Geometry: final body of the model. Coordinates: model frame, mm. A direction names the side the tool comes from. Coordinates: 2 decimals unless noted, no trailing zeros. Loops run counter-clockwise (first coordinate to the right, second up) from the corner with the lowest first, then second, coordinate; pieces in that order, holes last. Notation, with made-up numbers: M 23,42 L 34,42 A8 ccw 34,52 Z; hole C 64.25,-30 d3. An arc over 180 degrees is marked long. Write each question's results on one line, items separated by ' | '. Start each with the question number.
from build123d import *

# Parameters (mm, degrees)
F1_DEPTH  = 29
F0_W      = 28.9777747887
F0_H      = 95.25
F2_DEPTH  = 29
F5_DEPTH  = 3
F6_R      = 2.5
F7_D      = 3.2639
F10_R     = 2.5
F9_W      = 60
F9_H      = 26
F11_DEPTH = 97.505434954
F16_DEPTH = 0.5
F19_DEPTH = 0.5
F22_DEPTH = 0.5
F23_D     = 6.7564


# Not quite as in the source:
# - a feature names something its author has since deleted; it is built from what else it names


with BuildPart() as f1:
    # F0 (on Front) → F1 (new body)
    with BuildSketch(Plane.XZ):
        Polygon((28.9777747887, 7.7645713531), (0, 0), (28.9777747887, 0), align=None)
    extrude(amount=F1_DEPTH)

    # F0 (on Front) → F2 (join)
    with BuildSketch(Plane.XZ):
        Polygon((28.9777747887, 7.7645713531), (0, 0), (28.9777747887, 0), align=None)
        with Locations((14.4888873943, -47.625)):
            Rectangle(F0_W, F0_H)
    extrude(amount=F2_DEPTH)

    # F4 (on face) → F5 (join)
    with BuildSketch(Plane(origin=(0, 0, -95.25), x_dir=(1, 0, 0), z_dir=(0, 0, -1))):
        Polygon((0, 29), (14.4888873943, 29), (28.9777747887, 29), (28.9777747887, 34), (0, 34), align=None)
        Polygon((28.9777747887, 0), (14.4888873943, 0), (0, 0), (0, -5), (28.9777747887, -5), align=None)
    extrude(amount=-F5_DEPTH)

    # F6
    f6_edges = [f1.edges().sort_by_distance(p)[0] for p in [
        (28.977775, -34, -93.75),
        (0, -34, -93.75),
    ]]
    fillet(f6_edges, radius=F6_R)

    # F7 (through all)
    with Locations(Plane(origin=(0, 0, -95.25), x_dir=(1, 0, 0), z_dir=(0, 0, -1))):
        with Locations((2.5, 31.5), (14.4888873943, 31.5), (26.4777747887, 31.5), (2.5, -2.5), (14.4888873943, -2.5), (26.4777747887, -2.5)):
            Hole(F7_D / 2)

    # F10
    f10_edges = [f1.edges().sort_by_distance(p)[0] for p in [
        (28.977775, 5, -93.75),
        (0, 5, -93.75),
    ]]
    fillet(f10_edges, radius=F10_R)

    # F9 (on offset) → F11 (cut, through all)
    with BuildSketch(Plane(origin=(0.5176380902, 0, -1.9318516526), x_dir=(0.9659258263, 0, 0.2588190451), z_dir=(-0.2588190451, 0, 0.9659258263))):
        with Locations((-0.5358983849, -14.5)):
            Rectangle(F9_W, F9_H)
    extrude(amount=-F11_DEPTH, mode=Mode.SUBTRACT)

    # F15 (on plane+point) → F16 (join, symmetric)
    with BuildSketch(Plane.YZ.offset(20.4833310915)):
        Polygon((-29, -92.25), (-29, 5.4884920243), (-34, -92.25), align=None)
        Polygon((5, -92.25), (0, 5.4884920243), (0, -92.25), align=None)
    extrude(amount=F16_DEPTH, both=True)

    # F18 (on plane+point) → F19 (join, symmetric)
    with BuildSketch(Plane.YZ.offset(8.4944436972)):
        Polygon((5, -92.25), (0, 2.2760793288), (0, -92.25), align=None)
        Polygon((-34, -92.25), (-29, -92.25), (-29, 2.2760793288), align=None)
    extrude(amount=F19_DEPTH, both=True)

    # F21 (on plane+point) → F22 (join, symmetric)
    with BuildSketch(Plane.YZ.offset(14.4888873943)):
        Polygon((-27.5, 1.8117333157), (-27.5, -95.25), (-19.5, 1.8117333157), align=None)
        Polygon((-1.5, 1.8117333157), (-9.5, 1.8117333157), (-1.5, -95.25), align=None)
    extrude(amount=F22_DEPTH, both=True)

    # F23 (through all)
    with Locations(Plane(origin=(0, 0, 0), x_dir=(0.9659258263, 0, 0.2588190451), z_dir=(-0.2588190451, 0, 0.9659258263))):
        with Locations((15, -14.5)):
            Hole(F23_D / 2)


solid = f1.part
Item 1: Set-up query: faces 1 (the flat face through (24, -32, -92.25)), 2 (the flat face through (20.983, 1, -64)), 3 (the flat face through (20.49, 2.535, -44.065)), 4 (the flat face through (19.983, -30, -64)), 5 (the flat face through (19, -27.5, -47)). Return all of +Z, -Z, +X, -X, +Y, -Y with unobstructed straight access to the full face (end or side cutting, diameter ignored); none if empty.
Item 2: Ray query, L1, parallel to X at y = -31.5, z = -94.3; L2, parallel to Y at x = 2.5, z = -94.3; L3, parallel to Y at x = 7.25, z = -79.5. Return the intervals inside material, ascending. Write a range as [from, to].
Item 3: Contact query for flat-ended pins moving along their axis: P1, Ø2, axis at x = 11, y = -19, coming from the -Z side; P2, Ø5.5, axis at x = 27, y = 3, coming from the +Z side; P3, Ø1, axis at x = 17.5, y = -15, coming from the +Z side. Output: stop coordinate, or through.
Item 4: Pull-direction query (X, two-part tool) for faces 6 (the flat face through (20.983, -30, -64)), 7 (the flat face through (14, 0, -43)), 8 (the flat face through (8.487, 2.535, -45.649)); classes: released by +X, released by -X, zero draft, split by the parting line, or undercut.
Item 5: Section B-B, the plane y = -22.5. Return loops of the section in (x, z), plus the area to 3 significant figures.
Solutions:
1) face 1: +Z, +X, -Y | face 2: +Z, +X, +Y | face 3: +Z, +X, -X, +Y | face 4: +Z, -Y | face 5: -Z, +X
2) L1: x = [0, 0.87], [4.13, 12.86], [16.12, 24.85], [28.11, 28.98] | L2: y = [-34, -33.13], [-29.87, -27.5], [-1.5, 0.87], [4.13, 5] | L3: y = [-29, -27.5], [-1.5, 0]
3) P1: stops at z = 0.61 | P2: stops at z = -92.25 | P3: stops at z = 4.82
4) face 6: released by +X | face 7: undercut | face 8: zero draft
5) outline: M 0,-2.07 L 13.99,1.68 L 13.99,-34.59 L 14.99,-34.59 L 14.99,1.81 L 14.49,1.81 L 28.98,5.69 L 28.98,7.76 L 0,0 Z | area: 96.4 mm²
